```python
from build123d import *

# Parameters (mm, degrees)
SKETCH1_R           = 2.38
BOSS_EXTRUDE1_DEPTH = 6.35
FILLET1_R           = 2


with BuildPart() as part:
    # Sketch1 → Boss-Extrude1 (new body)
    with BuildSketch(Plane(origin=(0, 0, 0), x_dir=(1, 0, 0), z_dir=(0, 1, 0))):
        Polygon((-20, 12.5), (20, 12.5), (30, -12.5), (-30, -12.5), align=None)
        with Locations((-13.209810235, -3.549051176)):
            Circle(SKETCH1_R, mode=Mode.SUBTRACT)
        with Locations((13.209810235, -3.549051176)):
            Circle(SKETCH1_R, mode=Mode.SUBTRACT)
    extrude(amount=BOSS_EXTRUDE1_DEPTH)

    # Fillet1
    fillet1_edges = [part.edges().sort_by_distance(p)[0] for p in [
        (-20, 3.175, -12.5),
        (20, 3.175, -12.5),
        (30, 3.175, 12.5),
        (-30, 3.175, 12.5),
    ]]
    fillet(fillet1_edges, radius=FILLET1_R)


solid = part.part
```
Part model, mm, in its own coordinate system. Coordinates: 2 decimals unless noted, no trailing zeros. Write each loop counter-clockwise with the first axis right and the second up, starting at its lowest first coordinate (ties: lowest second). Pieces come first, ordered by that corner, then holes.
Item 1: Probe line 1 (X direction, y = 1.75, z = 5.25); line 2 (Z direction, x = -12, y = 4.25); line 3 (X direction, y = 0.75, z = -7). List the from-to ranges inside material, lowest first.
Item 2: Slice it at D-D (x = 21.5). Write the cut outline in (y, z), and give its area (3 significant figures).
Item 3: Slice it at C-C (y = 1). Write the cut outline in (x, z).
Item 4: Slice it at A-A (x = 14). Write the cut outline in (y, z), and give its area (3 significant figures).
Item 5: Slice it at B-B (z = -4.75). Write the cut outline in (x, y), and give its area (3 significant figures).
Item 6: Pin check, flat tip, straight feed: pin 1 (1.5 mm diameter, centred on y = 3, z = 0.5, fed in from -X). Stop position of the tip, or through.
Item 7: Mould opens along X. For faces 1 (the face through (-11.01, 3.13, 4.46)), 2 (the face through (28.717, 3.219, 11.599)), 3 (the face through (0, 0, 0)) say: released by +X, released by -X, zero draft, split by the parting line, or undercut.
Results found:
1. line 1: x = -27.1 to -14.87, -11.55 to 11.55, 14.87 to 27.1
1. line 2: z = -12.5 to 1.5, 5.6 to 12.5
1. line 3: x = -22.2 to 22.2
2. outline: (0, -8.75) - (6.35, -8.75) - (6.35, 12.5) - (0, 12.5) - close
2. area: 135 mm2
3. outline: (-28.9, 9.76) - (-20.5, -11.24) arc R2 ccw to (-18.65, -12.5) - (18.65, -12.5) arc R2 ccw to (20.5, -11.24) - (28.9, 9.76) arc R2 ccw to (27.05, 12.5) - (-27.05, 12.5) arc R2 ccw to start; hole circle Ø4.76 at (-13.21, 3.55); hole circle Ø4.76 at (13.21, 3.55)
4. outline: (0, -12.5) - (6.35, -12.5) - (6.35, 1.3) - (0, 1.3) - close; (0, 5.79) - (6.35, 5.79) - (6.35, 12.5) - (0, 12.5) - close
4. area: 130 mm2
5. outline: (-23.1, 0) - (23.1, 0) - (23.1, 6.35) - (-23.1, 6.35) - close
5. area: 293 mm2
6. pin 1: stops at x = -25.5
7. face 1: undercut
7. face 2: released by +X
7. face 3: zero draft
